```python
from build123d import *

# Parameters (mm, degrees)
SKETCH2_R              = 3.175
CUT_EXTRUDE1_DEPTH     = 6.35
CUT_EXTRUDE2_START     = 6.35
CUT_EXTRUDE2_OUTLINE_R = 1.75
CUT_EXTRUDE2_DEPTH     = 19.05
CUT_EXTRUDE3_DEPTH     = 7.62
CUT_EXTRUDE4_DEPTH     = 44.994090512


# Read off the part's stored shape, not the designer's step: Cut-Extrude2
with BuildPart() as part:
    # Sketch1 → Revolve1 (revolve)
    with BuildSketch(Plane.XY, mode=Mode.PRIVATE) as revolve1_sk:
        Polygon((0, 33.02), (0, 25.4), (7.62, 25.4), (5.08, 33.02), align=None)
        Polygon((0, 25.4), (0, 12.7), (25.4, 12.7), (25.4, 20.32), (24.13, 20.32), (24.13, 24.13), (25.4, 24.13), (25.4, 25.4), (7.62, 25.4), align=None)
        Polygon((0, 12.7), (0, 0), (25.4, 0), (25.4, 1.27), (24.13, 1.27), (24.13, 5.08), (25.4, 5.08), (25.4, 12.7), align=None)
    revolve(revolve1_sk.sketch.rotate(Axis((0, 25.4, 0), (0, -1, 0)), 180), axis=Axis((0, 25.4, 0), (0, -1, 0)))

    # Sketch2 → Cut-Extrude1 (cut)
    with BuildSketch(Plane(origin=(0, 0, 0), x_dir=(-1, 0, 0), z_dir=(0, -1, 0))):
        with Locations(Location((0, 0, 0), (0, 0, 180))):
            Circle(SKETCH2_R)
    extrude(amount=-CUT_EXTRUDE1_DEPTH, mode=Mode.SUBTRACT)

    # Cut-Extrude2 outline → Cut-Extrude2 (cut)
    with BuildSketch(Plane(origin=(0, 0, 0), x_dir=(1, 0, 0), z_dir=(0, 1, 0)).offset(CUT_EXTRUDE2_START)):
        Circle(CUT_EXTRUDE2_OUTLINE_R)
    extrude(amount=CUT_EXTRUDE2_DEPTH, mode=Mode.SUBTRACT)

    # Sketch3 → Cut-Extrude3 (cut)
    with BuildSketch(Plane(origin=(0, 33.02, 0), x_dir=(1, 0, 0), z_dir=(0, 1, 0))):
        with BuildLine():
            Line((2.155261469, 1.778), (-2.155261469, 1.778))
            ThreePointArc((-2.155261469, 1.778), (-2.794, 0), (-2.155261469, -1.778))
            Line((-2.155261469, -1.778), (2.155261469, -1.778))
            ThreePointArc((2.155261469, -1.778), (2.629471101, -0.944625708), (2.794, 0))
            ThreePointArc((2.794, 0), (2.629471101, 0.944625708), (2.155261469, 1.778))
        make_face()
    extrude(amount=-CUT_EXTRUDE3_DEPTH, mode=Mode.SUBTRACT)

    # Sketch4 → Cut-Extrude4 (cut, through all)
    with BuildSketch(Plane(origin=(0, 25.4, 0), x_dir=(1, 0, 0), z_dir=(0, 1, 0))):
        with BuildLine():
            ThreePointArc((-5.331998267, 5.443729832), (-2.354709497, 7.247050654), (1.113933099, 7.538139893))
            Line((1.113933099, 7.538139893), (4.66583568, 18.469771991))
            ThreePointArc((4.66583568, 18.469771991), (-5.886773743, 18.117626635), (-14.630999948, 12.199850021))
            Line((-14.630999948, 12.199850021), (-5.331998267, 5.443729832))
        make_face()
        with BuildLine():
            Line((-16.123974489, -10.144946855), (-6.824972808, -3.388826666))
            ThreePointArc((-6.824972808, -3.388826666), (-7.62, 0), (-6.824972808, 3.388826666))
            Line((-6.824972808, 3.388826666), (-16.123974489, 10.144946855))
            ThreePointArc((-16.123974489, 10.144946855), (-19.05, 0), (-16.123974489, -10.144946855))
        make_face()
        with BuildLine():
            Line((4.66583568, -18.469771991), (1.113933099, -7.538139893))
            ThreePointArc((1.113933099, -7.538139893), (-2.354709497, -7.247050654), (-5.331998267, -5.443729832))
            Line((-5.331998267, -5.443729832), (-14.630999948, -12.199850021))
            ThreePointArc((-14.630999948, -12.199850021), (-5.886773743, -18.117626635), (4.66583568, -18.469771991))
        make_face()
        with BuildLine():
            Line((19.007619525, -1.27), (7.513421325, -1.27))
            ThreePointArc((7.513421325, -1.27), (6.164709497, -4.478923622), (3.529616651, -6.753236728))
            Line((3.529616651, -6.753236728), (7.081519231, -17.684868825))
            ThreePointArc((7.081519231, -17.684868825), (15.411773743, -11.197309056), (19.007619525, -1.27))
        make_face()
        with BuildLine():
            ThreePointArc((3.529616651, 6.753236728), (6.164709497, 4.478923622), (7.513421325, 1.27))
            Line((7.513421325, 1.27), (19.007619525, 1.27))
            ThreePointArc((19.007619525, 1.27), (15.411773743, 11.197309056), (7.081519231, 17.684868825))
            Line((7.081519231, 17.684868825), (3.529616651, 6.753236728))
        make_face()
    extrude(amount=-CUT_EXTRUDE4_DEPTH, mode=Mode.SUBTRACT)


solid = part.part
```
Can you work these out from the model? Positions are in its coordinate system, mm. A direction names the side the tool comes from. Round coordinates to 2 decimals unless told otherwise and drop trailing zeros. Loops run counter-clockwise (first coordinate to the right, second up) from the corner with the lowest first, then second, coordinate; pieces in that order, holes last. Notation, with made-up numbers: M -32.75,68.25 L -27.75,68.25 A5 cw -27.75,75.25 Z; hole C 27.25,-26 d6. An arc over 180 degrees is marked long. Answer as a JSON object with one key per item and string values. Group by question number.
Q1. Imagine slicing it at C-C, the plane x = 0. Count the separate pieces of the cut face and the enclosed holes in it, then the cut area to 3 significant figures.
Q2. Imagine slicing it at D-D, the plane y = 13.5. Please give me the cut outline in (x, z), then the cut area to 3 significant figures.
Q3. Imagine slicing it at B-B, the plane z = 16.5. Please give me the cut outline in (x, y).
Q4. Imagine slicing it at A-A, the plane y = 3.5. Please give me the cut outline in (x, z) (3 decimals), then the cut area to 3 significant figures.
Q5. On a 3-axis mill with a long thin cutter (end or side, diameter ignored), from which of +Z, -Z, +X, -X, +Y, -Y can I reach the whole of each face in a straight line? I mean faces 1 (the cylindrical face through (-23.016, 3.202, -7.248)), 2 (the cylindrical face through (6.136, 12.878, -4.519)), 3 (the cylindrical face through (-2.794, 29.263, -0.027)), 4 (the cylindrical face through (1.5, 3.1, -2.8)). Say none if no direction works.
Q6. We'd pull the mould along X, two halves only. Please class faces 5 (the flat face through (5, 0, 0)), 6 (the flat face through (2, 25.4, 0)), 7 (the cylindrical face through (-11.721, 12.807, 22.534)): +X half, -X half, draft (parallel to the pull), parting line (faces both ways), or undercut.
Q7. Please list where these lines run through material, in increasing order: L1, parallel to Y at x = -20, z = -15; L2, parallel to Z at x = 0, y = 21; L3, parallel to Z at x = 0, y = 13.75.
Q8. Will these pins go through, and if not, where does the flat tip stop? pin 1 (3 mm diameter, centred on y = 8.5, z = 8, fed in from -X); pin 2 (5 mm diameter, centred on y = 28.5, z = -5.5, fed in from -X); pin 3 (5.5 mm diameter, centred on x = 0, z = 0, fed in from -Y); pin 4 (1.8 mm diameter, centred on x = 0.5, z = 0.5, fed in from +Y).
Findings:
{
 "1": {"separate pieces": "4", "enclosed holes": "0", "area": "653 mm2"},
 "2": {"outline": "C 0,0 d50.8; hole M -16.12,-10.14 L -6.82,-3.39 A7.62 cw -6.82,3.39 L -16.12,10.14 A19.05 ccw Z; hole M -14.63,-12.2 A19.05 ccw 4.67,-18.47 L 1.11,-7.54 A7.62 cw -5.33,-5.44 Z; hole M -14.63,12.2 L -5.33,5.44 A7.62 cw 1.11,7.54 L 4.67,18.47 A19.05 ccw Z; hole C 0,0 d3.5; hole M 3.53,-6.75 L 7.08,-17.68 A19.05 ccw 19.01,-1.27 L 7.51,-1.27 A7.62 cw Z; hole M 3.53,6.75 A7.62 cw 7.51,1.27 L 19.01,1.27 A19.05 ccw 7.08,17.68 Z", "area": "1,200 mm2"},
 "3": {"outline": "M -19.31,0 L -9.52,0 L -9.52,25.4 L -19.31,25.4 L -19.31,24.13 L -17.61,24.13 L -17.61,20.32 L -19.31,20.32 L -19.31,5.08 L -17.61,5.08 L -17.61,1.27 L -19.31,1.27 Z; M 4.03,0 L 6.7,0 L 6.7,25.4 L 4.03,25.4 Z; M 9.52,0 L 19.31,0 L 19.31,1.27 L 17.61,1.27 L 17.61,5.08 L 19.31,5.08 L 19.31,20.32 L 17.61,20.32 L 17.61,24.13 L 19.31,24.13 L 19.31,25.4 L 9.52,25.4 Z"},
 "4": {"outline": "C 0,0 d48.26; hole M -16.124,-10.145 L -6.825,-3.389 A7.62 cw -6.825,3.389 L -16.124,10.145 A19.05 ccw Z; hole M -14.631,-12.2 A19.05 ccw 4.666,-18.47 L 1.114,-7.538 A7.62 cw -5.332,-5.444 Z; hole M -14.631,12.2 L -5.332,5.444 A7.62 cw 1.114,7.538 L 4.666,18.47 A19.05 ccw Z; hole C 0,0 d6.35; hole M 3.53,-6.753 L 7.082,-17.685 A19.05 ccw 19.008,-1.27 L 7.513,-1.27 A7.62 cw Z; hole M 3.53,6.753 A7.62 cw 7.513,1.27 L 19.008,1.27 A19.05 ccw 7.082,17.685 Z", "area": "985 mm2"},
 "5": {"face 1": "none", "face 2": "+Y, -Y", "face 3": "+Y", "face 4": "-Y"},
 "6": {"face 5": "draft", "face 6": "undercut", "face 7": "parting line"},
 "7": {"L1": "y = 0 to 1.27, 5.08 to 20.32, 24.13 to 25.4", "L2": "z = -24.13 to -19.05, -7.62 to -1.75, 1.75 to 7.62, 19.05 to 24.13", "L3": "z = -25.4 to -19.05, -7.62 to -1.75, 1.75 to 7.62, 19.05 to 25.4"},
 "8": {"pin 1": "stops at x = -24.55", "pin 2": "stops at x = -6.16", "pin 3": "stops at y = 6.35", "pin 4": "passes through"}
}
